Design review of the part built by this model. Coordinates are the model's own, in mm. Face numbers are marked on the shaded views. A direction names the side the tool comes from. Round coordinates to 2 decimals unless told otherwise and drop trailing zeros. Loops run counter-clockwise (first coordinate to the right, second up) from the corner with the lowest first, then second, coordinate; pieces in that order, holes last. Notation, with made-up numbers: (59, 43.5) - (84, 43.5) arc R32 cw to (84, 77.5) - close; hole circle Ø9 at (45.25, -28.5). An arc over 180 degrees is marked (long way). Use one line per item in the form item = value. Start each with the question number.
(1) Machinability: for the marked faces 1, 2 and 3, which of the approach directions +Z, -Z, +X, -X, +Y, -Y give a long, thin tool a straight path to every point of the face, cutting with its end or side? Answer none if there is none.
(2) For pin 1 (3.5 mm diameter, centred on y = 4.5, z = 1, fed in from -X); pin 2 (3.5 mm diameter, centred on x = 13, y = 7, fed in from -Z); pin 3 (3 mm diameter, centred on y = 8.5, z = -9, fed in from +X); pin 4 (1.3 mm diameter, centred on x = 5.5, y = 6, fed in from -Z), all flat-tipped, find the tip position at first contact; note any pin that passes through.
(3) Wall thickness on probe 1 along Y at (x, z) = (13.8, -6.7); probe 2 along Y at (x, z) = (5.5, -13.1); probe 3 along Z at (x, y) = (-4.5, 8.5): over which ranges is each line inside the solid? List them lowest first. Write a range as [from, to].
(4) We need section A-A, the plane x = -13.8. Write out the cut boundary in (y, z).
(5) We need section B-B, the plane x = 5.5. Write out the cut boundary in (y, z), then the cut area to 3 significant figures.
(6) We need section C-C, the plane y = 1.25. Write out the cut boundary in (x, z).
(7) We need section D-D, the plane z = 8.25. Write out the cut boundary in (x, y), then the cut area to 3 significant figures.
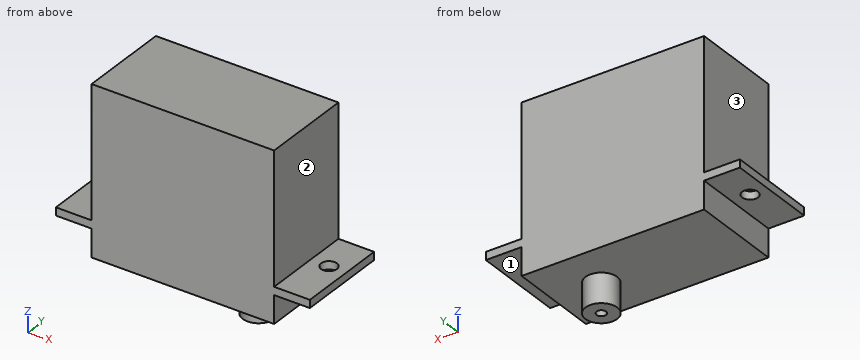
from build123d import *

# Parameters (mm, degrees)
SKETCH1_W           = 23
SKETCH1_H           = 21
BOSS_EXTRUDE1_DEPTH = 11.6
SKETCH2_W           = 1
SKETCH2_H           = 11.6
BOSS_EXTRUDE2_DEPTH = 4.5
SKETCH3_R           = 2
SKETCH3_R_2         = 0.6
BOSS_EXTRUDE3_DEPTH = 3.7
SKETCH4_R           = 1
CUT_EXTRUDE1_DEPTH  = 5


with BuildPart() as part:
    # Sketch1 → Boss-Extrude1 (new body)
    with BuildSketch(Plane(origin=(0, 0, 0), x_dir=(1, 0, 0), z_dir=(0, 1, 0))):
        Rectangle(SKETCH1_W, SKETCH1_H)
    extrude(amount=BOSS_EXTRUDE1_DEPTH)

    # Sketch2 → Boss-Extrude2 (add)
    with BuildSketch(Plane(origin=(11.5, 0, 0), x_dir=(0, 0, -1), z_dir=(1, 0, 0))):
        with Locations((6.5, 5.8)):
            Rectangle(SKETCH2_W, SKETCH2_H)
    boss_extrude2 = extrude(amount=BOSS_EXTRUDE2_DEPTH)

    # Mirror1: Boss-Extrude2 across plane
    add(boss_extrude2.mirror(Plane(origin=(0, 0, 0), x_dir=(0, 0, 1), z_dir=(1, 0, 0))))

    # Sketch3 → Boss-Extrude3 (add)
    with BuildSketch(Plane(origin=(0, 0, -10.5), x_dir=(-1, 0, 0), z_dir=(0, 0, -1))):
        with Locations((-5.5, 5.8)):
            Circle(SKETCH3_R)
        with Locations((-5.5, 5.8)):
            Circle(SKETCH3_R_2, mode=Mode.SUBTRACT)
    extrude(amount=BOSS_EXTRUDE3_DEPTH)

    # Sketch4 → Cut-Extrude1 (cut)
    with BuildSketch(Plane(origin=(0, 0, -7), x_dir=(-1, 0, 0), z_dir=(0, 0, -1))):
        with Locations((-13.8, 6.6)):
            Circle(SKETCH4_R)
        with Locations((13.8, 6.6)):
            Circle(SKETCH4_R)
    extrude(amount=-CUT_EXTRUDE1_DEPTH, mode=Mode.SUBTRACT)


solid = part.part
Data:
q1.face_1 = -Z, +X, +Y, -Y
q1.face_2 = +Z, +X, +Y, -Y
q1.face_3 = +Z, -X, +Y, -Y
q2.pin_1 = -11.5
q2.pin_2 = -10.5
q2.pin_3 = 11.5
q2.pin_4 = -14.2
q3.probe_1 = [0, 5.6], [7.6, 11.6]
q3.probe_2 = [3.8, 5.2], [6.4, 7.8]
q3.probe_3 = [-10.5, 10.5]
q4.outline = (0, -7) - (5.6, -7) - (5.6, -6) - (0, -6) - close; (7.6, -7) - (11.6, -7) - (11.6, -6) - (7.6, -6) - close
q5.outline = (0, -10.5) - (3.8, -10.5) - (3.8, -14.2) - (5.2, -14.2) - (5.2, -10.5) - (6.4, -10.5) - (6.4, -14.2) - (7.8, -14.2) - (7.8, -10.5) - (11.6, -10.5) - (11.6, 10.5) - (0, 10.5) - close
q5.area = 254 mm^2
q6.outline = (-16, -7) - (-11.5, -7) - (-11.5, -10.5) - (11.5, -10.5) - (11.5, -7) - (16, -7) - (16, -6) - (11.5, -6) - (11.5, 10.5) - (-11.5, 10.5) - (-11.5, -6) - (-16, -6) - close
q7.outline = (-11.5, 0) - (11.5, 0) - (11.5, 11.6) - (-11.5, 11.6) - close
q7.area = 267 mm^2
